The drawing under review shows one solid part. Ordinate dimensions are in mm from its lowest x, y, z. A direction names the side the tool comes from. Coordinates: 2 decimals unless noted, no trailing zeros. Order: outer loops, then holes, each group sorted by start corner. A loop starts at its lowest first (then second) coordinate and runs counter-clockwise, first axis right, second up.
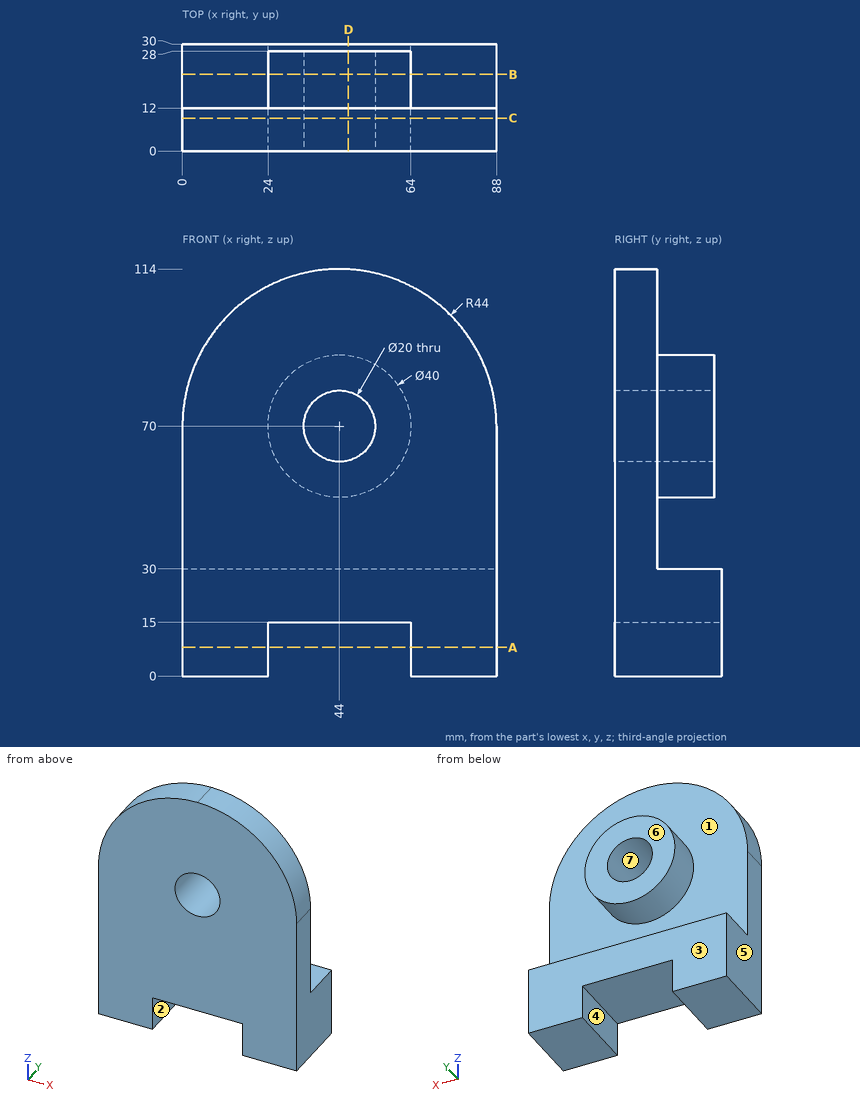
1. To check wall thickness, follow L1, parallel to X at y = 9.5, z = 70; L2, parallel to X at y = 12.25, z = 70; L3, parallel to Y at x = 73, z = 103. State the ranges of each line that lie inside material, in increasing order.
Answer below:
L1: x = 0 to 34, 54 to 88
L2: x = 24 to 34, 54 to 64
L3: y = 0 to 12
2. Machinability: for the marked faces 1, 2 and 3, which of the approach directions +Z, -Z, +X, -X, +Y, -Y give a long, thin tool a straight path to every point of the face, cutting with its end or side? Answer none if there is none.
Answer below:
face 1: +Y
face 2: -Z, +Y, -Y
face 3: +Z, -Z, +X, -X, +Y
3. The part is to be moulded in two halves that separate along X. For the marked faces 4, 5, 6 and 7, say which applies: +X half, -X half, draft (parallel to the pull), parting line (faces both ways), or undercut.
Answer below:
face 4: undercut
face 5: -X half
face 6: draft
face 7: undercut
4. Take a section at B-B, the plane y = 21.5. Give the boundary of the cut face in (x, z), plus the area to 3 significant figures.
Answer below:
outline: (0, 0) - (24, 0) - (24, 15) - (64, 15) - (64, 0) - (88, 0) - (88, 30) - (0, 30) - close; circle Ø40 at (44, 70); hole circle Ø20 at (44, 70)
area: 2,980 mm2
5. Take a section at A-A, the plane z = 8. Give the boundary of the cut face in (x, y), plus the area to 3 significant figures.
Answer below:
outline: (0, 0) - (24, 0) - (24, 30) - (0, 30) - close; (64, 0) - (88, 0) - (88, 30) - (64, 30) - close
area: 1,440 mm2
6. Take a section at D-D, the plane x = 46.5. Give the boundary of the cut face in (y, z), plus the area to 3 significant figures.
Answer below:
outline: (0, 15) - (30, 15) - (30, 30) - (12, 30) - (12, 50.16) - (28, 50.16) - (28, 60.32) - (0, 60.32) - close; (0, 79.68) - (28, 79.68) - (28, 89.84) - (12, 89.84) - (12, 113.93) - (0, 113.93) - close
area: 1,550 mm2
7. Take a section at C-C, the plane y = 9.25. Give the boundary of the cut face in (x, z).
Answer below:
outline: (0, 0) - (24, 0) - (24, 15) - (64, 15) - (64, 0) - (88, 0) - (88, 70) arc R44 ccw to (44, 114) arc R44 ccw to (0, 70) - close; hole circle Ø20 at (44, 70)
8. Clearance check with flat-ended pins moving along their axes: pin 1 Ø1 at (x, y) = (38.5, 27) entering from -Z; pin 2 Ø6 at (x, z) = (20, 86) entering from +Y; pin 3 Ø5 at (x, z) = (63.5, 76.5) entering from +Y; pin 4 Ø16 at (x, z) = (44, 70) entering from +Y. State where each tip first meets the part, or that it passes through.
Answer below:
pin 1: stops at z = 15
pin 2: stops at y = 12
pin 3: stops at y = 28
pin 4: passes through
